Work out the finished part from the listing and answer in its coordinate system (mm). Face numbers are marked on the shaded views. A direction names the side the tool comes from. Round coordinates to 2 decimals unless told otherwise and drop trailing zeros. Write each loop counter-clockwise with the first axis right and the second up, starting at its lowest first coordinate (ties: lowest second). Pieces come first, ordered by that corner, then holes. Notation, with made-up numbers: (-20, -10.5) - (25, -10.5) arc R18 cw to (25, -3.5) - close; hole circle Ø9 at (17.25, -37). An arc over 180 degrees is marked (long way). Write item = value, one per line. Start each with the question number.
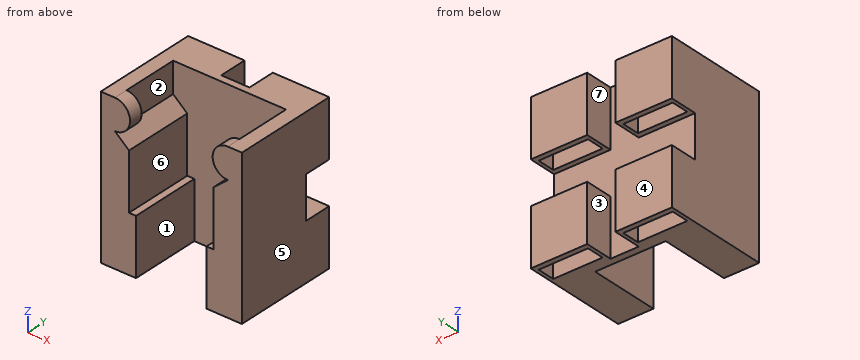
from build123d import *

# Parameters (mm, degrees)
F0_W      = 20
F0_H      = 22
F1_DEPTH  = 11
F3_DEPTH  = 10
F5_DEPTH  = 2
F6_W      = 8
F6_H      = 8
F7_DEPTH  = 4
F8_W      = 7
F8_H      = 2.5
F9_DEPTH  = 25
F11_W     = 8
F11_H     = 4
F12_DEPTH = 1
F10_W     = 8
F10_H     = 4
F13_DEPTH = 1


with BuildPart() as f1:
    # F0 (on Front) → F1 (new body)
    with BuildSketch(Plane.XZ):
        Rectangle(F0_W, F0_H)
    extrude(amount=F1_DEPTH)

    # F2 (on face) → F3 (cut)
    with BuildSketch(Plane.XZ.offset(11)):
        Polygon((8, 6.704264), (8, 11), (-8, 11), (-8, 6.704264), (-6, 5), (-6, -3), (-5, -3), (-5, -11), (5, -11), (5, -3), (6, -3), (6, 5), align=None)
    extrude(amount=-F3_DEPTH, mode=Mode.SUBTRACT)

    # F4 (on face) → F5 (join)
    with BuildSketch(Plane.XZ.offset(11)):
        with BuildLine():
            Line((-8, 11), (-8, 6.704264))
            ThreePointArc((-8, 6.704264), (-5.852132, 8.852132), (-8, 11))
        make_face()
        with BuildLine():
            ThreePointArc((8, 11), (5.852132, 8.852132), (8, 6.704264))
            Line((8, 6.704264), (8, 11))
        make_face()
    extrude(amount=-F5_DEPTH)

    # F6 (on face) → F7 (join)
    with BuildSketch(Plane(origin=(0, 0, 0), x_dir=(-1, 0, 0), z_dir=(0, 1, 0))):
        with Locations((-6, 7)):
            Rectangle(F6_W, F6_H)
        with Locations((6, 7)):
            Rectangle(F6_W, F6_H)
        with Locations((-6, -7)):
            Rectangle(F6_W, F6_H)
        with Locations((6, -7)):
            Rectangle(F6_W, F6_H)
    extrude(amount=F7_DEPTH)

    # F8 (on face) → F9 (cut)
    with BuildSketch(Plane.XY.offset(11)):
        with Locations((-6, 2)):
            Rectangle(F8_W, F8_H)
        with Locations((6, 2)):
            Rectangle(F8_W, F8_H)
    extrude(amount=-F9_DEPTH, mode=Mode.SUBTRACT)

    # F11 (on face) → F12 (join)
    with BuildSketch(Plane.XY.offset(-3)):
        with Locations((6, 2)):
            Rectangle(F11_W, F11_H)
        with Locations((-6, 2)):
            Rectangle(F11_W, F11_H)
    extrude(amount=-F12_DEPTH)

    # F10 (on face) → F13 (join)
    with BuildSketch(Plane.XY.offset(11)):
        with Locations((6, 2)):
            Rectangle(F10_W, F10_H)
        with Locations((-6, 2)):
            Rectangle(F10_W, F10_H)
    extrude(amount=-F13_DEPTH)


solid = f1.part
1. Find section C-C on y = 2. Give the number of separate pieces and of enclosed holes in the cut face, plus the area to 3 significant figures.
2. Consider line 1 (X direction, y = 1.5, z = -7.5); line 2 (X direction, y = 2.75, z = -3.5); line 3 (Y direction, x = 4.75, z = 6.25). Determine where each line is inside the solid, lowest interval first.
3. Find section B-B on z = -8. Give the vertices of the cut face in (x, y), plus the area to 3 significant figures.
4. Find section D-D on x = -6.75. Give the vertices of the cut face in (y, z).
5. Each of these flat-tipped pins is pushed along its axis until it touches: pin 1 (1.2 mm diameter, centred on x = 5.5, y = 2, fed in from -Z); pin 2 (1 mm diameter, centred on x = 3.5, z = -8, fed in from -Y). Where does it stop, or does it pass through?
6. Which of the six approach directions +Z, -Z, +X, -X, +Y, -Y give full straight-line access (tool end or side, diameter ignored) to the marked faces 1, 2 and 3?
7. Find section A-A on y = -8.5. Give the vertices of the cut face in (x, z).
8. For a pull along X with two mould halves and no side action, classify the marked faces 4, 5, 6 and 7 as released by +X, released by -X, zero draft, split by the parting line, or undercut.
Answer key:
q1.separate_pieces = 4
q1.enclosed_holes = 0
q1.area = 60.0 mm²
q2.line_1 = -10 to -9.5, -2.5 to -2, 2 to 2.5, 9.5 to 10
q2.line_2 = -10 to -2, 2 to 10
q2.line_3 = -1 to 0.75, 3.25 to 4
q3.outline = (-10, -11) - (-5, -11) - (-5, -1) - (5, -1) - (5, -11) - (10, -11) - (10, 4) - (2, 4) - (2, 0) - (-2, 0) - (-2, 4) - (-10, 4) - close; hole (-9.5, 0.75) - (-2.5, 0.75) - (-2.5, 3.25) - (-9.5, 3.25) - close; hole (2.5, 0.75) - (9.5, 0.75) - (9.5, 3.25) - (2.5, 3.25) - close
q3.area = 149 mm²
q4.outline = (-11, -11) - (0.75, -11) - (0.75, -4) - (3.25, -4) - (3.25, -11) - (4, -11) - (4, -3) - (0, -3) - (0, 3) - (0.75, 3) - (0.75, 10) - (3.25, 10) - (3.25, 3) - (4, 3) - (4, 11) - (-1, 11) - (-1, 5.64) - (-11, 5.64) - close; (-11, 7.11) - (-9, 7.11) - (-9, 10.6) - (-11, 10.6) - close
q5.pin_1 = -4
q5.pin_2 = -1
q6.face_1 = +Z, -Z, -Y
q6.face_2 = +Z
q6.face_3 = +Z, -Z, +Y
q7.outline = (-10, -11) - (-5, -11) - (-5, -3) - (-6, -3) - (-6, 5) - (-8, 6.7) - (-8, 11) - (-10, 11) - close; (5, -11) - (10, -11) - (10, 11) - (8, 11) - (8, 6.7) - (6, 5) - (6, -3) - (5, -3) - close
q8.face_4 = zero draft
q8.face_5 = released by +X
q8.face_6 = undercut
q8.face_7 = undercut
